Solid Edge part; units mm, degrees
sketch "Sketch1" plane through (0, 0, 0) normal (0, -1, 0) x (1, 0, 0)
  line L0 (-20, -10) -> (20, -10)
  line L1 (20, -10) -> (20, 10)
  line L2 (20, 10) -> (-20, 10)
  line L3 (-20, 10) -> (-20, -10)
  dimension "D1" = 20
  dimension "D2" = 20
extrude "Protrusion1" add sketch "Sketch1" along normal mid plane 1000
sketch "Sketch2" plane through (0, -500, 0) normal (0, -1, 0) x (1, 0, 0)
  line L0 (-20, -3) -> (-18.5, -3)
  line L1 (-18.5, -3) -> (-18.5, -6.15)
  line L2 (-18.5, -6.15) -> (-17, -6.15)
  line L3 (-14.3, -3.45) -> (-17, -6.15)
  line L4 (-14.3, -3.45) -> (-14.3, 3.45)
  line L5 (-14.3, 3.45) -> (-17, 6.15)
  line L6 (-18.5, 6.15) -> (-17, 6.15)
  line L7 (-18.5, 6.15) -> (-18.5, 3)
  line L8 (-18.5, 3) -> (-20, 3)
  line L9 (-20, 3) -> (-20, -3)
  dimension "D1" = 20
  dimension "D2" = 14.3
  dimension "D3" = 18.5
  dimension "D4" = 20
extrude "Cutout1" cut sketch "Sketch2" against normal through all
fillet "Verrundung_1" radius 1.5 4 edges at (20, 0, 10) (-20, 0, 10) (20, 0, -10) (-20, 0, -10)
pattern_circular "Pattern1" count 4 over 360 about axis through (-10, -500, 0) along (0, -1, 0) of "Cutout1"
fillet "Round1" [suppressed]
fillet "Round2" [suppressed]
fillet "Round3" [suppressed]
mirror "Mirror1" about plane through (0, 0, 0) normal (1, 0, 0) of "Cutout1", "Pattern1"
fillet "Round4" [suppressed]
fillet "Round5" [suppressed]
fillet "Round6" [suppressed]
fillet "Round7" [suppressed]
sketch "Sketch3" plane through (0, -500, 0) normal (0, -1, 0) x (-1, 0, 0)
  line L0 (-3, 8.5) -> (3, 8.5)
  line L1 (3, 8.5) -> (3, -8.5)
  line L2 (3, -8.5) -> (-3, -8.5)
  line L3 (-3, -8.5) -> (-3, 8.5)
extrude "Cutout9" cut sketch "Sketch3" against normal through all
hole "Hole1" at (-10, -500, 0) direction (0, 1, 0) diameter 5.5 end up to next
hole "Hole2" at (10, -500, 0) direction (0, 1, 0) diameter 5.5 end up to next
sketch "Sketch4" plane through (0, -500, 0) normal (0, -1, 0) x (1, 0, 0)
  line L0 (-18.5, 3) -> (-20, 4.5)
  line L1 (-20, 4.5) -> (-20, 3)
  line L2 (-20, 3) -> (-18.5, 3)
  line L3 (-18.5, -3) -> (-20, -4.5)
  line L4 (-20, -4.5) -> (-20, -3)
  line L5 (-20, -3) -> (-18.5, -3)
  line L6 (18.5, 3) -> (20, 4.5)
  line L7 (20, 4.5) -> (20, 3)
  line L8 (20, 3) -> (18.5, 3)
  line L9 (18.5, -3) -> (20, -3)
  line L10 (20, -4.5) -> (20, -3)
  line L11 (20, -4.5) -> (18.5, -3)
extrude "Cutout10" cut sketch "Sketch4" against normal through all
sketch "Sketch5" plane through (0, 0, -10) normal (0, 0, -1) x (0, 1, 0)
  line L0 (-480, 5) -> (-480, -20)
  line L1 (-480, -20) -> (-500, -20)
  line L2 (-500, -20) -> (-500, 5)
  line L3 (-480, 5) -> (-500, 5)
  dimension "D1" = 480
  dimension "D2" = 500
extrude "Cutout11" cut sketch "Sketch5" against normal through all
mirror "Mirror2" about plane through (0, 0, 0) normal (0, -1, 0) of "Cutout11"
Design review of the part built by this model. Coordinates are the model's own, in mm. A direction names the side the tool comes from. Give positions to 0.01 mm unless a question says otherwise; leave off trailing zeros. Use CSV: the item, a comma, the result in double quotes. Start each with the question number.
1. Add section A-A (y = 382). Count the separate pieces of the cut face and the enclosed holes in it, plus the area to 3 significant figures.
2. Wall thickness on L1, parallel to X at y = -168, z = 0; L2, parallel to X at y = -186, z = 9.25; L3, parallel to Z at x = -6.5, y = -346: over which ranges is each line inside the solid? List them lowest first.
3. Insertion check: P1, Ø5, axis at x = -4, z = 4, coming from the -Y side; P2, Ø3, axis at y = 55.5, z = 0, coming from the +X side; P3, Ø5.5, axis at x = -10, y = 97.5, coming from the -Z side; P4, Ø8, axis at x = 1.5, z = -0.5, coming from the +Y side. Each pin has a flat end and moves straight along its axis. Give the tip position at first contact, or say it passes through.
4. Machinability: for faces 1 (the flat face through (-9, 480, -3)), 2 (the flat face through (-7, -480, -2)), which of the approach directions +Z, -Z, +X, -X, +Y, -Y give a long, thin tool a straight path to every point of the face, cutting with its end or side? Answer none if there is none.
Results found:
1,separate pieces,"1"
1,enclosed holes,"3"
1,area,"272 mm²"
2,L1,"x = -14.3 to -12.75, -7.25 to -5.7, 5.7 to 7.25, 12.75 to 14.3"
2,L2,"x = -19.8 to -13, -7 to 7, 13 to 19.8"
2,L3,"z = -10 to -8.5, -4.35 to 4.35, 8.5 to 10"
3,P1,"stops at y = -480"
3,P2,"stops at x = 14.3"
3,P3,"stops at z = -4.3"
3,P4,"passes through"
4,face 1,"+Z, -Z, -X, +Y"
4,face 2,"+Z, -Z, -X, -Y"
